```python
from build123d import *

# Parameters (mm, degrees)
BOSS_EXTRUDE1_DEPTH      = 30
BOSS_EXTRUDE1_DEPTH_BACK = 30
CUT_EXTRUDE1_DEPTH       = 13
BOSS_EXTRUDE2_START      = -8
BOSS_EXTRUDE2_DEPTH      = 8
BOSS_EXTRUDE3_DEPTH      = 5
SKETCH5_R                = 5
BOSS_EXTRUDE4_DEPTH      = 8
CUT_EXTRUDE2_DEPTH       = 9
SKETCH7_R                = 5
CUT_EXTRUDE3_DEPTH       = 104.596573302
SKETCH8_R                = 5
CUT_EXTRUDE4_DEPTH       = 96.032889044
CUT_EXTRUDE5_DEPTH       = 109.310895112


with BuildPart() as part:
    # Sketch1 → Boss-Extrude1 (new, two sides: drawn at the far end of the back side and taken through both)
    with BuildSketch(Plane.XY.offset(-BOSS_EXTRUDE1_DEPTH_BACK)):
        with BuildLine():
            Line((-65, 9.998359599), (-65, 0))
            Line((-65, 0), (65, 0))
            Line((65, 0), (65, 47.5))
            Line((65, 47.5), (25, 47.5))
            Line((25, 47.5), (25, 62.5))
            Line((25, 62.5), (-35, 62.5))
            Line((-35, 62.5), (-35, 39.686269666))
            ThreePointArc((-35, 39.686269666), (-43.896848552, 18.675004673), (-65, 9.998359599))
        make_face()
    extrude(amount=BOSS_EXTRUDE1_DEPTH + BOSS_EXTRUDE1_DEPTH_BACK)

    # Sketch2 → Cut-Extrude1 (cut)
    with BuildSketch(Plane.XY.offset(30)):
        with BuildLine():
            Line((-35, 59.686269666), (-35.00136791, 39.71351659))
            ThreePointArc((-35.00136791, 39.71351659), (-36.817077306, 29.717837367), (-41.86475429, 20.901298318))
            ThreePointArc((-41.86475429, 20.901298318), (-15.306099587, 36.200543555), (-35, 59.686269666))
        make_face()
    extrude(amount=-CUT_EXTRUDE1_DEPTH, mode=Mode.SUBTRACT)

    # Sketch3 → Boss-Extrude2 (add)
    with BuildSketch(Plane.XY.offset(30).offset(BOSS_EXTRUDE2_START)):
        with BuildLine():
            Line((-65, 9.998359599), (-65, 15))
            ThreePointArc((-65, 15), (-54.833160932, 17.160661495), (-46.42368968, 23.269169331))
            ThreePointArc((-46.42368968, 23.269169331), (-44.219987435, 21.937644338), (-41.863489254, 20.900254001))
            ThreePointArc((-41.863489254, 20.900254001), (-52.211827427, 12.860341399), (-65, 9.998359599))
        make_face()
    extrude(amount=BOSS_EXTRUDE2_DEPTH)

    # Sketch4 → Boss-Extrude3 (add)
    with BuildSketch(Plane.XY.offset(17)):
        with BuildLine():
            Line((-35, 47.186269666), (-35, 39.686269666))
            ThreePointArc((-35, 39.686269666), (-35.235297751, 35.936269666), (-35.9375, 32.245094104))
            ThreePointArc((-35.9375, 32.245094104), (-27.514720556, 39.216597822), (-35, 47.186269666))
        make_face()
    extrude(amount=BOSS_EXTRUDE3_DEPTH)

    # Sketch5 → Boss-Extrude4 (add)
    with BuildSketch(Plane.XY.offset(22)):
        with Locations(Location((-35, 39.686269666, 0), (0, 0, 265.219808153))):
            Circle(SKETCH5_R)
    extrude(amount=BOSS_EXTRUDE4_DEPTH)

    # Sketch6 → Cut-Extrude2 (cut)
    with BuildSketch(Plane.XY.offset(30)):
        with BuildLine():
            Line((65, 47.5), (45, 47.5))
            Line((45, 47.5), (45, 39.686269666))
            ThreePointArc((45, 39.686269666), (50.857864376, 25.544134042), (65, 19.686269666))
            Line((65, 19.686269666), (65, 39.686269666))
            Line((65, 39.686269666), (65, 47.5))
        make_face()
    extrude(amount=-CUT_EXTRUDE2_DEPTH, mode=Mode.SUBTRACT)

    # Sketch7 → Cut-Extrude3 (cut, through all)
    with BuildSketch(Plane.XY.offset(21)):
        with Locations((55, 40)):
            Circle(SKETCH7_R)
    extrude(amount=-CUT_EXTRUDE3_DEPTH, mode=Mode.SUBTRACT)

    # Sketch8 → Cut-Extrude4 (cut, through all)
    with BuildSketch(Plane(origin=(0, 62.5, 0), x_dir=(1, 0, 0), z_dir=(0, 1, 0))):
        with Locations(Location((-25, 5, 0), (0, 0, 180))):
            Circle(SKETCH8_R)
    extrude(amount=-CUT_EXTRUDE4_DEPTH, mode=Mode.SUBTRACT)

    # Sketch9 → Cut-Extrude5 (cut, through all)
    with BuildSketch(Plane.XY.offset(30)):
        with BuildLine():
            Line((25, 0), (50, 0))
            Line((50, 0), (43.562275488, 6.437724512))
            ThreePointArc((43.562275488, 6.437724512), (40.679372543, 7.859414913), (37.526741582, 7.232317625))
            Line((37.526741582, 7.232317625), (25, 0))
        make_face()
    extrude(amount=-CUT_EXTRUDE5_DEPTH, mode=Mode.SUBTRACT)


solid = part.part
```
CAD build for the part. Positions are in the model's coordinates, mm. A direction names the side the tool comes from. Round coordinates to 2 decimals unless told otherwise and drop trailing zeros. Loops run counter-clockwise (first coordinate to the right, second up) from the corner with the lowest first, then second, coordinate; pieces in that order, holes last. Notation, with made-up numbers: M 76.25,-5 L 114.25,-5 A4 cw 114.25,1 Z; hole C 52,-3 d1. An arc over 180 degrees is marked long. Use a Markdown table: item, result. Add a question column.
(1) Cut at D-D (y = 58). Give the cut face in (x, z).
(2) Flat gauge pins, fed straight in: pin 1 (9 mm diameter, centred on x = 55, y = 40, fed in from +Z); pin 2 (2.5 mm diameter, centred on y = 45, z = 27.5, fed in from +X); pin 3 (12 mm diameter, centred on y = 48, z = -15.5, fed in from -X); pin 4 (7.5 mm diameter, centred on y = 57, z = 11.5, fed in from +X). Where does each tip first touch, or does it go through?
(3) Drill centre lines: line 1 (Z direction, x = -25, y = 40.5); line 2 (Z direction, x = -25, y = 19); line 3 (Y direction, x = -21.5, z = 19). Where is each one in solid material? Low to high.
(4) Cut at C-C (x = -25). Give the cut face in (y, z), and give its area (3 significant figures).
(5) Cut at B-B (y = 27). Give the cut face in (x, z).
(6) Cut at A-A (x = 55). Give the cut face in (y, z).
(7) Which spindle directions (+Z, -Z, +X, -X, +Y, -Y) get a long thin tool onto all of the face, cutting with end or side? Do faces 1 (the face through (47, 3, 0)), 2 (the face through (25, 55, 0)), 3 (the face through (-39.613, 37.757, 25.944)), 4 (the face through (-35, 51, -7)). Say none if no direction does.
(8) Pull direction X, two halves, no side cores. Call faces 5 (the face through (45, 47.5, 0)), 6 (the face through (-44.252, 21.954, 25.944)), 7 (the face through (45, 44, 26)), 8 (the face through (-65, 6, 0)): +X half, -X half, draft (parallel to the pull), parting line (faces both ways), or undercut.
Geometry says:
| question | item | result |
|---|---|---|
| 1 | outline | M -35,-30 L 25,-30 L 25,30 L -26.96,30 L -26.96,17 L -35,17 Z; hole C -25,-5 d10 |
| 2 | pin 1 | passes through |
| 2 | pin 2 | stops at x = 45 |
| 2 | pin 3 | stops at x = -35 |
| 2 | pin 4 | stops at x = 25 |
| 3 | line 1 | z = -30 to -10, 0 to 17 |
| 3 | line 2 | z = -30 to -10, 0 to 30 |
| 3 | line 3 | y = 0 to 24.93, 54.44 to 62.5 |
| 4 | outline | M 0,-30 L 62.5,-30 L 62.5,-10 L 0,-10 Z; M 0,0 L 62.5,0 L 62.5,30 L 57.01,30 L 57.01,17 L 22.37,17 L 22.37,30 L 0,30 Z |
| 4 | area | 2,670 mm² |
| 5 | outline | M -37.96,-30 L 65,-30 L 65,21 L 49.54,21 L 49.54,30 L -19.54,30 L -19.54,17 L -37.96,17 Z; hole C -25,-5 d10 |
| 6 | outline | M 0,-30 L 35,-30 L 35,21 L 22.37,21 L 22.37,30 L 0,30 Z; M 45,-30 L 47.5,-30 L 47.5,21 L 45,21 Z |
| 7 | face 1 | +Z, -Z, -Y |
| 7 | face 2 | +Z, -Z, +X, +Y |
| 7 | face 3 | +Z |
| 7 | face 4 | -Z, -X, +Y |
| 8 | face 5 | draft |
| 8 | face 6 | undercut |
| 8 | face 7 | +X half |
| 8 | face 8 | -X half |
